Autodesk Inventor part; units mm, degrees
ref_plane "YZ Plane" through (0, 0, 0) normal (1, 0, 0) x (0, 1, 0)
ref_plane "XZ Plane" through (0, 0, 0) normal (0, 1, 0) x (-1, 0, 0)
ref_plane "XY Plane" through (0, 0, 0) normal (0, 0, 1) x (1, 0, 0)
sketch "Sketch1" plane through (0, 0, 0) normal (0, 1, 0) x (-1, 0, 0)
  line L0 (0, 0) -> (11.5, 0)
  line L1 (11.5, 0) -> (11.5, -12)
  line L2 (11.5, -12) -> (0, -12)
  line L3 (0, -12) -> (0, 0)
  line L4 (0, -12) -> (5.2, -12)
  line L5 (5.2, -12) -> (5.2, 0)
  line L6 (5.2, 0) -> (0, 0)
  line L7 (0, 0) -> (0, -12)
  line L8 (0, 0) -> (2.3, 0)
  line L9 (2.3, 0) -> (2.3, -12)
  line L10 (2.3, -12) -> (0, -12)
  line L11 (0, -12) -> (0, 0)
  line L12 (2.3, 0) -> (2.3, -3)
  line L13 (2.3, -3) -> (2.3, -9)
  circle A0 centre (2.3, -3) radius 1
  circle A1 centre (2.3, -9) radius 1
  dimension "d0" = 11.5
  dimension "d1" = 12
  dimension "d2" = 5.2
  dimension "d3" = 2.3
  dimension "d4" = 3
  dimension "d5" = 6
  dimension "d6" = 2
  dimension "d7" = 2
extrude "Extrusion1" add sketch "Sketch1" along normal blind 0.13 contours L0 L9 A0 A1 L2 L3 | L0 L5 L2 L9 A1 A0 | L0 L1 L2 L5
bend part "Bend Part1" radius 0.5 angle 90 line through (-5.2, 0, -12) along (0, 0, 1) centre toward (0, 1, 0) moving side (-1, 0, 0) both sides no
properties part number "Clmap for sample mount for new Leica System"
Geometry check sheet. Reference: the model listing, model coordinates, mm. Give positions to 0.01 mm unless a question says otherwise; leave off trailing zeros. Order: outer loops, then holes, each group sorted by start corner. A loop starts at its lowest first (then second) coordinate and runs counter-clockwise, first axis right, second up. Notation, with made-up numbers: (74.25, -16) - (116.25, -16) arc R19 cw to (116.25, 1) - close; hole circle Ø1 at (78.25, 73). An arc over 180 degrees is marked (long way). Use one line per item in the form item = value.
1) Material ranges on probe 1 along Z at (x, y) = (-2.3, 0.05), recorded low to high. Write a range as from..to.
Working result:
probe_1 = -12..-10, -8..-4, -2..0
2) Sectioned sample at B-B (x = -2.3). Record the boundary of the cut face in (y, z).
Working result:
outline = (0, -12) - (0.13, -12) - (0.13, -10) - (0, -10) - close; (0, -8) - (0.13, -8) - (0.13, -4) - (0, -4) - close; (0, -2) - (0.13, -2) - (0.13, 0) - (0, 0) - close
3) Sectioned sample at C-C (z = -7.5). Record the boundary of the cut face in (x, y).
Working result:
outline = (-5.7, 0.5) arc R0.5 ccw to (-5.2, 0) - (0, 0) - (0, 0.13) - (-5.2, 0.13) arc R0.37 cw to (-5.57, 0.5) - (-5.57, 6.01) - (-5.7, 6.01) - close
4) Sectioned sample at A-A (z = -9). Record the boundary of the cut face in (x, y), and give its area (3 significant figures).
Working result:
outline = (-5.7, 0.5) arc R0.5 ccw to (-5.2, 0) - (-3.3, 0) - (-3.3, 0.13) - (-5.2, 0.13) arc R0.37 cw to (-5.57, 0.5) - (-5.57, 6.01) - (-5.7, 6.01) - close; (-1.3, 0) - (0, 0) - (0, 0.13) - (-1.3, 0.13) - close
area = 1.22 mm^2
5) Depth check by flat-ended pin: pin 1 Ø3 at (x, y) = (-2, 0.5) entering from +Z; pin 2 Ø1.6 at (x, z) = (-2, -4) entering from +Y; pin 3 Ø1 at (y, z) = (4.5, -8) entering from +X; pin 4 Ø1.5 at (x, y) = (-3, 2.5) entering from +Z. Enter the tip coordinate at first touch or a pass-through.
Working result:
pin_1 = 0
pin_2 = 0.13
pin_3 = -5.57
pin_4 = through
6) Sectioned sample at D-D (x = -2.9). Record the boundary of the cut face in (y, z), and give its area (3 significant figures).
Working result:
outline = (0, -12) - (0.13, -12) - (0.13, -9.8) - (0, -9.8) - close; (0, -8.2) - (0.13, -8.2) - (0.13, -3.8) - (0, -3.8) - close; (0, -2.2) - (0.13, -2.2) - (0.13, 0) - (0, 0) - close
area = 1.14 mm^2
